Design review of the part built by this model. Coordinates are the model's own, in mm. Coordinates: 2 decimals unless noted, no trailing zeros. Write each loop counter-clockwise with the first axis right and the second up, starting at its lowest first coordinate (ties: lowest second). Pieces come first, ordered by that corner, then holes. Notation, with made-up numbers: (61, 50) -> (85, 50) arc R26 cw to (85, 64) -> close; hole circle Ø8 at (-34.5, 6). An arc over 180 degrees is marked (long way). One line per question, with ' | ' between items. Start each with the question number.
Q1. Add section C-C on z = 11. State the section outline as (x, y) points, and give its area (3 significant figures).
Q2. Add section B-B on y = -304.5. State the section outline as (x, z) points.
Q3. Add section A-A on x = -13. State the section outline as (y, z) points.
Q4. For P1, Ø6, axis at y = -50, z = 0, coming from the -X side; P2, Ø7.5, axis at y = -50, z = 0, coming from the -X side, all flat-tipped, find the tip position at first contact; note any pin that passes through.
Q5. Wall thickness on probe 1 along Y at (x, z) = (19, 0); probe 2 along Z at (x, y) = (-19, -50); probe 3 along X at (y, z) = (-487, -14.5): over which ranges is each line inside the solid? List them lowest first.
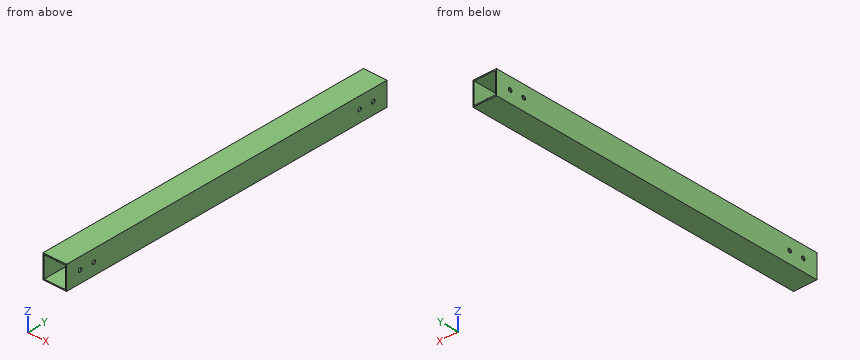
from build123d import *

# Parameters (mm, degrees)
SKETCH_W    = 40
SKETCH_H    = 40
SKETCH_W_2  = 36
SKETCH_H_2  = 36
PAD_DEPTH   = 588
SKETCH001_R = 3.3
HOLE_DEPTH  = 40.001


with BuildPart() as part:
    # Sketch → Pad (new body)
    with BuildSketch(Plane.XZ):
        Rectangle(SKETCH_W, SKETCH_H)
        Rectangle(SKETCH_W_2, SKETCH_H_2, mode=Mode.SUBTRACT)
    extrude(amount=PAD_DEPTH)

    # Sketch001 → Hole (cut, through all)
    with BuildSketch(Plane(origin=(20, 0, 0), x_dir=(0, 0, 1), z_dir=(1, 0, 0))):
        with Locations((0, 25)):
            Circle(SKETCH001_R)
        with Locations((0, 50)):
            Circle(SKETCH001_R)
        with Locations((0, 563)):
            Circle(SKETCH001_R)
        with Locations((0, 538)):
            Circle(SKETCH001_R)
    extrude(amount=-HOLE_DEPTH, mode=Mode.SUBTRACT)


solid = part.part
Output values:
1) outline: (-20, -588) -> (-18, -588) -> (-18, 0) -> (-20, 0) -> close; (18, -588) -> (20, -588) -> (20, 0) -> (18, 0) -> close | area: 2,350 mm2
2) outline: (-20, -20) -> (20, -20) -> (20, 20) -> (-20, 20) -> close; hole (-18, -18) -> (18, -18) -> (18, 18) -> (-18, 18) -> close
3) outline: (-588, -20) -> (0, -20) -> (0, -18) -> (-588, -18) -> close; (-588, 18) -> (0, 18) -> (0, 20) -> (-588, 20) -> close
4) P1: passes through | P2: stops at x = -20
5) probe 1: y = -588 to -566.3, -559.7 to -541.3, -534.7 to -53.3, -46.7 to -28.3, -21.7 to 0 | probe 2: z = -20 to -3.3, 3.3 to 20 | probe 3: x = -20 to -18, 18 to 20
